For this review, take the finished solid that the model builds, in its own axes (mm). Face numbers are marked on the shaded views. A direction names the side the tool comes from. Coordinates: 2 decimals unless noted, no trailing zeros. Write each loop counter-clockwise with the first axis right and the second up, starting at its lowest first coordinate (ties: lowest second). Pieces come first, ordered by that corner, then holes.
1) Insertion check: P1, Ø1.5, axis at x = 34.5, z = 14.5, coming from the +Y side; P2, Ø8, axis at x = -10.5, z = 31.5, coming from the +Y side; P3, Ø6, axis at y = 26, z = 10.5, coming from the +X side (3 decimals). Each pin has a flat end and moves straight along its axis. Give the tip position at first contact, or say it passes through.
2) To check wall thickness, follow line 1 along Z through (x, y) = (49, 10.5); line 2 along Y through (x, z) = (69, -13.5); line 3 along Y through (x, z) = (-81.5, -26). State the ranges of each line that lie inside material, in increasing order.
3) We need section A-A on z = -15.5. Write out the cut boundary in (x, y).
4) For the marked faces 1 and 2, list the 3-axis set-ups (+Z, -Z, +X, -X, +Y, -Y) from which the entire face can be reached by the end or side of a thin tool; tool diameter is ignored.
5) We need section C-C on x = -29. Write out the cut boundary in (y, z).
6) We need section D-D on z = 27.5. Write out the cut boundary in (x, y), then the cut area to 3 significant figures.
7) Mouldability with a two-part tool opening along Y and no side actions: class the marked faces 3, 4 and 5 as pulls with the +Y half, pulls with the -Y half, needs draft (parallel to the pull), parting line crosses it, or undercut.
8) We need section B-B on y = 9. Write out the cut boundary in (x, z).
from build123d import *

# Parameters (mm, degrees)
SKETCH_1_W      = 30
SKETCH_1_H      = 10
SKETCH_1_W_2    = 70
SKETCH_1_W_3    = 10
EXTRUDE_1_DEPTH = 100


with BuildPart() as part:
    # Эскиз1 → Бобышка-Вытянуть1 (new, symmetric)
    with BuildSketch(Plane(origin=(0, 0, 0), x_dir=(0, 0, -1), z_dir=(1, 0, 0))):
        Polygon((-5, 65), (-5, 5), (5, 5), (5, 55), (5, 65), align=None)
        with Locations((20, 60)):
            Rectangle(SKETCH_1_W, SKETCH_1_H)
        Rectangle(SKETCH_1_W_2, SKETCH_1_H)
        with Locations((30, 10)):
            Rectangle(SKETCH_1_W_3, SKETCH_1_H)
        with Locations((-30, 10)):
            Rectangle(SKETCH_1_W_3, SKETCH_1_H)
    extrude(amount=EXTRUDE_1_DEPTH, both=True)


solid = part.part
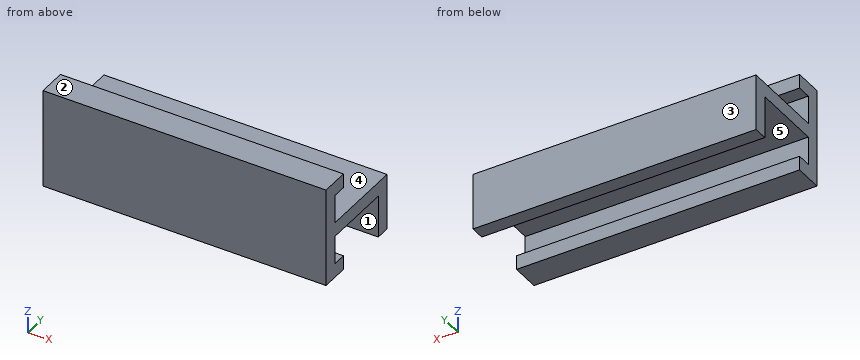
Result:
1. P1: stops at y = 5
1. P2: stops at y = 15
1. P3: passes through
2. line 1: z = -35 to -25, -5 to 5, 25 to 35
2. line 2: y = -5 to 5, 55 to 65
2. line 3: y = -5 to 15, 55 to 65
3. outline: (-100, -5) - (100, -5) - (100, 5) - (-100, 5) - close; (-100, 55) - (100, 55) - (100, 65) - (-100, 65) - close
4. face 1: -Z, +X, -X
4. face 2: +Z, +X, -X, +Y, -Y
5. outline: (-5, -35) - (15, -35) - (15, -25) - (5, -25) - (5, -5) - (55, -5) - (55, -35) - (65, -35) - (65, 5) - (5, 5) - (5, 25) - (15, 25) - (15, 35) - (-5, 35) - close
6. outline: (-100, -5) - (100, -5) - (100, 15) - (-100, 15) - close
6. area: 4,000 mm2
7. face 3: pulls with the +Y half
7. face 4: needs draft
7. face 5: undercut
8. outline: (-100, -35) - (100, -35) - (100, -25) - (-100, -25) - close; (-100, -5) - (100, -5) - (100, 5) - (-100, 5) - close; (-100, 25) - (100, 25) - (100, 35) - (-100, 35) - close
